Here's how the part is built. I have some questions about the finished solid (model axes, mm). A direction names the side the tool comes from. Round coordinates to 2 decimals unless told otherwise and drop trailing zeros. Order: outer loops, then holes, each group sorted by start corner. A loop starts at its lowest first (then second) coordinate and runs counter-clockwise, first axis right, second up. Notation, with made-up numbers: M 72,79.25 L 100,79.25 A27 cw 100,109.25 Z; hole C 38.5,82.25 d6. An arc over 180 degrees is marked long. Write item = value, one per line. Start each with the question number.
Item 1: I want a section at A-A, the plane x = 53.5. List the corners of the cut face in (y, z) for me.
Item 2: Please list where these lines run through material, in increasing order: L1, parallel to X at y = 28, z = 8.5; L2, parallel to Y at x = -43, z = 22; L3, parallel to Z at x = -120.65, y = 53.75.
Item 3: We'd pull the mould along Z, two halves only. Please class faces 6 (the face through (-123.57, 53.93, 12.15)), 7 (the face through (2, 6, 0)), 8 (the face through (77.216, 31, 13)): pulls with the +Z half, pulls with the -Z half, needs draft (parallel to the pull), parting line crosses it, or undercut.
Item 4: I want a section at C-C, the plane z = 17.5. List the corners of the cut face in (x, y) for me.
Item 5: I want a section at D-D, the plane x = -106.5. List the corners of the cut face in (y, z) for me, plus the area to 3 significant figures.
Item 6: For faces 1 (the face through (101.6, 19, 13)), 2 (the face through (-101.6, 19, 13)), 3 (the face through (118.456, 53.931, 14.212)), 4 (the face through (-1, 12.7, 13)), 5 (the face through (-2, 6, 25.4)), which set-ups out of +Z, -Z, +X, -X, +Y, -Y let a thin tool reach every point of the face, with its end or its side?
Item 7: I'm going to push flat-ended pins straight in: P1, Ø10, axis at y = 48, z = 3.5, coming from the +X side; P2, Ø12.5, axis at y = 15, z = 19, coming from the +X side; P3, Ø9.5, axis at x = 120.61, z = 12.24, coming from the -Y side; P4, Ø7.5, axis at y = 35.5, z = 12, coming from the -X side. Where does each tip first touch, or does it pass through?
Item 8: I want a section at B-B, the plane y = 35. List the corners of the cut face in (x, z) for me, plus the area to 3 significant figures.
```python
from build123d import *

# Parameters (mm, degrees)
F0_W     = 203.2
F0_H     = 25.4
F1_DEPTH = 25.4
F2_W     = 24.3940738201
F2_H     = 25.4
F2_W_2   = 24.384
F3_DEPTH = 38.1
F4_W     = 38.1
F4_H     = 25.4
F4_W_2   = 203.1179050207
F5_DEPTH = 6.35
F6_R     = 2.921
F7_DEPTH = 25.4
F8_R     = 2.921
F9_DEPTH = 25.4


with BuildPart() as f1:
    # F0 (on Top) → F1 (new body)
    with BuildSketch(Plane.XY):
        Rectangle(F0_W, F0_H)
    extrude(amount=F1_DEPTH)

    # F2 (on face) → F3 (join)
    with BuildSketch(Plane(origin=(0, 12.7, 0), x_dir=(-1, 0, 0), z_dir=(0, 1, 0))):
        with Locations((89.4029630899, 12.7)):
            Rectangle(F2_W, F2_H)
        with Locations((-89.408, 12.7)):
            Rectangle(F2_W_2, F2_H)
    extrude(amount=F3_DEPTH)

    # F4 (on face) → F5 (join)
    with BuildSketch(Plane(origin=(0, 50.8, 0), x_dir=(-1, 0, 0), z_dir=(0, 1, 0))):
        with Locations((120.65, 12.7)):
            Rectangle(F4_W, F4_H)
        with Locations((0.0410474896, 12.7)):
            Rectangle(F4_W_2, F4_H)
        with Locations((-120.5679050207, 12.7)):
            Rectangle(F4_W, F4_H)
    extrude(amount=F5_DEPTH)

    # F6 (on face) → F7 (cut)
    with BuildSketch(Plane.XZ.offset(-50.8)):
        with Locations((-120.65, 12.0200840756)):
            Circle(F6_R)
    extrude(amount=-F7_DEPTH, mode=Mode.SUBTRACT)

    # F8 (on face) → F9 (cut)
    with BuildSketch(Plane.XZ.offset(-50.8)):
        with Locations((120.6089525104, 12.2376885265)):
            Circle(F8_R)
    extrude(amount=-F9_DEPTH, mode=Mode.SUBTRACT)


solid = f1.part
```
Filled in:
q1.outline = M -12.7,0 L 12.7,0 L 12.7,25.4 L -12.7,25.4 Z; M 50.8,0 L 57.15,0 L 57.15,25.4 L 50.8,25.4 Z
q2.L1 = -101.6 to -77.21, 77.22 to 101.6
q2.L2 = -12.7 to 12.7, 50.8 to 57.15
q2.L3 = 0 to 9.1, 14.94 to 25.4
q3.face_6 = undercut
q3.face_7 = pulls with the -Z half
q3.face_8 = needs draft
q4.outline = M -139.7,50.8 L -101.6,50.8 L -101.6,-12.7 L 101.6,-12.7 L 101.6,50.8 L 139.62,50.8 L 139.62,57.15 L -139.7,57.15 Z; hole M -77.21,12.7 L 77.22,12.7 L 77.22,50.8 L -77.21,50.8 Z
q5.outline = M 50.8,0 L 57.15,0 L 57.15,25.4 L 50.8,25.4 Z
q5.area = 161 mm^2
q6.face_1 = +Z, -Z, +X, -Y
q6.face_2 = +Z, -Z, -X, -Y
q6.face_3 = +Y, -Y
q6.face_4 = +Z, -Z
q6.face_5 = +Z, +X, -X, +Y, -Y
q7.P1 = 139.62
q7.P2 = 101.6
q7.P3 = 50.8
q7.P4 = -101.6
q8.outline = M -101.6,0 L -77.21,0 L -77.21,25.4 L -101.6,25.4 Z; M 77.22,0 L 101.6,0 L 101.6,25.4 L 77.22,25.4 Z
q8.area = 1,240 mm^2
